Verification items for the finished model (mm, model axes). Give positions to 0.01 mm unless a question says otherwise; leave off trailing zeros. Write each loop counter-clockwise with the first axis right and the second up, starting at its lowest first coordinate (ties: lowest second). Pieces come first, ordered by that corner, then holes. Notation, with made-up numbers: (64, 50.5) - (70, 50.5) arc R22 ccw to (70, 81.5) - close; hole circle Ø8 at (11.25, 8). An arc over 180 degrees is marked (long way). Answer as a JSON object with one key per item and string values. Group by question number.
Item 1: Sectioned sample at A-A, the plane x = 158. Record the boundary of the cut face in (y, z), and give its area (4 significant figures).
Item 2: Scan lines: line 1 along X through (y, z) = (-17, 4.35); line 2 along Y through (x, z) = (145.5, 1.2); line 3 along Y through (x, z) = (14.5, 2.75). Record each from-to range of solid material in increasing order. Write a range as [from, to].
Item 3: Go/stop test with flat-tipped pins: pin 1 (2.5 mm diameter, centred on x = 28.5, z = 3.5, fed in from +Y); pin 2 (1.5 mm diameter, centred on y = -16, z = 2, fed in from -X); pin 3 (1.5 mm diameter, centred on y = -31.5, z = 1.5, fed in from -X); pin 4 (1.5 mm diameter, centred on y = -147.5, z = 2.5, fed in from +X). Record where each tip stops, or that it passes through.
Item 4: Sectioned sample at B-B, the plane y = -145. Record the boundary of the cut face in (x, z).
```python
from build123d import *

# Parameters (mm, degrees)
F0_W     = 40
F0_H     = 7
F1_DEPTH = 5


with BuildPart() as f1:
    # F0 (on Top) → F1 (new body)
    with BuildSketch(Plane.XY):
        with BuildLine():
            Line((25, 0), (0, 0))
            Line((0, 0), (0, -25))
            Line((0, -25), (5, -25))
            Line((5, -25), (5, -38))
            Line((5, -38), (8.5, -38))
            ThreePointArc((8.5, -38), (10.692753, -35.101021), (14.156854, -34))
            Line((14.156854, -34), (19.156854, -34))
            Line((19.156854, -34), (19.156854, -46))
            Line((19.156854, -46), (14.156854, -46))
            ThreePointArc((14.156854, -46), (10.692753, -44.898979), (8.5, -42))
            Line((8.5, -42), (5, -42))
            Line((5, -42), (5, -55))
            Line((5, -55), (0, -55))
            Line((0, -55), (0, -140))
            Line((0, -140), (5, -140))
            Line((5, -140), (5, -153))
            Line((5, -153), (8.5, -153))
            ThreePointArc((8.5, -153), (10.692753, -150.101021), (14.156854, -149))
            Line((14.156854, -149), (19.156854, -149))
            Line((19.156854, -149), (19.156854, -161))
            Line((19.156854, -161), (14.156854, -161))
            ThreePointArc((14.156854, -161), (10.692753, -159.898979), (8.5, -157))
            Line((8.5, -157), (5, -157))
            Line((5, -157), (5, -170))
            Line((5, -170), (0, -170))
            Line((0, -170), (0, -194))
            Line((0, -194), (20, -194))
            Line((20, -194), (20, -201))
            Line((20, -201), (0, -201))
            Line((0, -201), (0, -300))
            Line((0, -300), (300, -300))
            Line((300, -300), (300, -201))
            Line((300, -201), (280, -201))
            Line((280, -201), (280, -194))
            Line((280, -194), (300, -194))
            Line((300, -194), (300, -170))
            Line((300, -170), (295, -170))
            Line((295, -170), (295, -157))
            Line((295, -157), (291.5, -157))
            ThreePointArc((291.5, -157), (289.307247, -159.898979), (285.843146, -161))
            Line((285.843146, -161), (280.843146, -161))
            Line((280.843146, -161), (280.843146, -149))
            Line((280.843146, -149), (285.843146, -149))
            ThreePointArc((285.843146, -149), (289.307247, -150.101021), (291.5, -153))
            Line((291.5, -153), (295, -153))
            Line((295, -153), (295, -140))
            Line((295, -140), (300, -140))
            Line((300, -140), (300, -55))
            Line((300, -55), (295, -55))
            Line((295, -55), (295, -42))
            Line((295, -42), (291.5, -42))
            ThreePointArc((291.5, -42), (289.307247, -44.898979), (285.843146, -46))
            Line((285.843146, -46), (280.843146, -46))
            Line((280.843146, -46), (280.843146, -34))
            Line((280.843146, -34), (285.843146, -34))
            ThreePointArc((285.843146, -34), (289.307247, -35.101021), (291.5, -38))
            Line((291.5, -38), (295, -38))
            Line((295, -38), (295, -25))
            Line((295, -25), (300, -25))
            Line((300, -25), (300, 0))
            Line((300, 0), (275, 0))
            Line((275, 0), (275, -5))
            Line((275, -5), (262, -5))
            Line((262, -5), (262, -8.5))
            ThreePointArc((262, -8.5), (264.898979, -10.692753), (266, -14.156854))
            Line((266, -14.156854), (266, -19.156854))
            Line((266, -19.156854), (254, -19.156854))
            Line((254, -19.156854), (254, -14.156854))
            ThreePointArc((254, -14.156854), (255.101021, -10.692753), (258, -8.5))
            Line((258, -8.5), (258, -5))
            Line((258, -5), (245, -5))
            Line((245, -5), (245, 0))
            Line((245, 0), (55, 0))
            Line((55, 0), (55, -5))
            Line((55, -5), (42, -5))
            Line((42, -5), (42, -8.5))
            ThreePointArc((42, -8.5), (44.898979, -10.692753), (46, -14.156854))
            Line((46, -14.156854), (46, -19.156854))
            Line((46, -19.156854), (34, -19.156854))
            Line((34, -19.156854), (34, -14.156854))
            ThreePointArc((34, -14.156854), (35.101021, -10.692753), (38, -8.5))
            Line((38, -8.5), (38, -5))
            Line((38, -5), (25, -5))
            Line((25, -5), (25, 0))
        make_face()
        with Locations((150, -197.5)):
            Rectangle(F0_W, F0_H, mode=Mode.SUBTRACT)
    extrude(amount=F1_DEPTH)


solid = f1.part
```
Geometry check:
{
 "1": {"outline": "(-300, 0) - (-201, 0) - (-201, 5) - (-300, 5) - close; (-194, 0) - (0, 0) - (0, 5) - (-194, 5) - close", "area": "1,465 mm^2"},
 "2": {"line 1": "[0, 34], [46, 254], [266, 300]", "line 2": "[-300, -201], [-194, 0]", "line 3": "[-300, -201], [-194, -161], [-149, -46], [-34, 0]"},
 "3": {"pin 1": "y = -5", "pin 2": "x = 0", "pin 3": "x = 5", "pin 4": "x = 295"},
 "4": {"outline": "(5, 0) - (295, 0) - (295, 5) - (5, 5) - close"}
}
